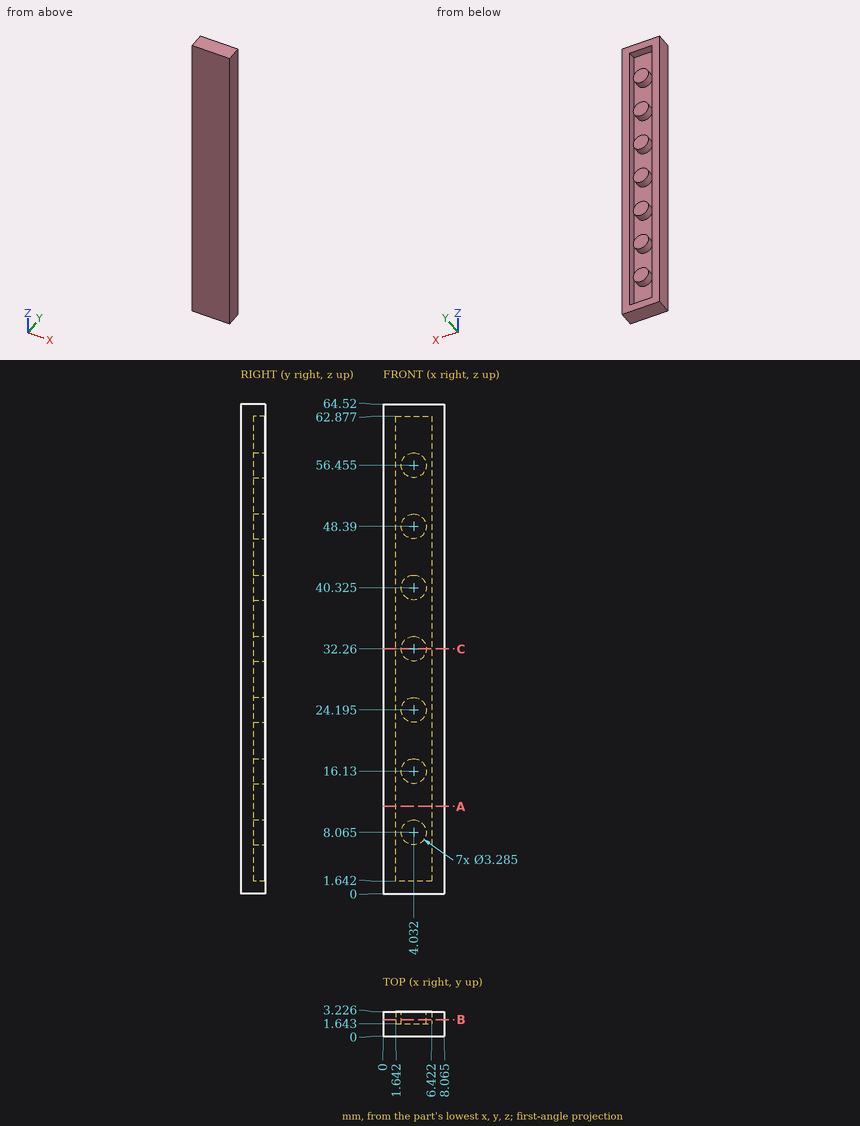
Input: dimensioned drawing with shaded views. Units: mm. Origin: part minimum x, y, z. Coordinates: 2 decimals unless noted, no trailing zeros. Loops run counter-clockwise (first coordinate to the right, second up) from the corner with the lowest first, then second, coordinate; pieces in that order, holes last. Notation, with made-up numbers: (38.5, -3) -> (75.5, -3) arc R8 ccw to (75.5, 5) -> close; hole circle Ø7 at (-19, 71.5). An arc over 180 degrees is marked (long way). One line per item, written item: value. Start each with the question number.
Q1. Line query: line 1 along Z through (x, y) = (2, 2.8); line 2 along X through (y, z) = (2.55, 38.5) (1 decimal); line 3 along X through (y, z) = (2.35, 55.5) (1 decimal). Output: solid intervals per line, ascending.
Q2. Section query B-B, the plane y = 2.15. Give the number of separate pieces and of enclosed holes in the cut face, and give its area (3 significant figures).
Q3. Section query A-A, the plane z = 11.5. Return the cut outline in (x, y) (1 decimal).
Q4. Section query C-C, the plane z = 32.26. Return the cut outline in (x, y) (1 decimal).
Results:
1. line 1: 0 to 1.64, 62.88 to 64.52
1. line 2: 0 to 1.6, 6.4 to 8.1
1. line 3: 0 to 1.6, 2.7 to 5.4, 6.4 to 8.1
2. separate pieces: 8
2. enclosed holes: 1
2. area: 287 mm^2
3. outline: (0, 0) -> (8.1, 0) -> (8.1, 3.2) -> (6.4, 3.2) -> (6.4, 1.6) -> (1.6, 1.6) -> (1.6, 3.2) -> (0, 3.2) -> close
4. outline: (0, 0) -> (8.1, 0) -> (8.1, 3.2) -> (6.4, 3.2) -> (6.4, 1.6) -> (5.7, 1.6) -> (5.7, 3.2) -> (2.4, 3.2) -> (2.4, 1.6) -> (1.6, 1.6) -> (1.6, 3.2) -> (0, 3.2) -> close
